The listing builds one solid part. Answer for the finished solid, in the listing's coordinates (mm). Face numbers are marked on the shaded views. A direction names the side the tool comes from. Coordinates: 2 decimals unless noted, no trailing zeros. Loops run counter-clockwise (first coordinate to the right, second up) from the corner with the lowest first, then second, coordinate; pieces in that order, holes last. Notation, with made-up numbers: (74, 23.5) - (133, 23.5) arc R11 ccw to (133, 33.5) - close; hole circle Ø2 at (-15.5, -30.5). An arc over 180 degrees is marked (long way). Return JSON: item names as keys, results as strings. Group by question number.
1. Which of the six approach directions +Z, -Z, +X, -X, +Y, -Y give full straight-line access (tool end or side, diameter ignored) to the marked faces 1 and 2?
2. Find the intervals of material crossed by line 1 along X through (y, z) = (19, -9); line 2 along Y through (x, z) = (2.15, 14.5); line 3 along Y through (x, z) = (-0.75, 16), in increasing order.
3. Section A-A (z = 8) is taken. Write down the section's boundary in (x, y).
4. Section B-B (y = 9.5) is taken. Write down the section's boundary in (x, z).
5. Each of these flat-tipped pins is pushed along its axis until it touches: P1, Ø9, axis at y = 10, z = 2.5, coming from the +X side; P2, Ø0.5, axis at x = -0.5, z = 4, coming from the +Y side; P3, Ø3, axis at y = 18, z = 15, coming from the -X side. Where does it stop, or does it pass through?
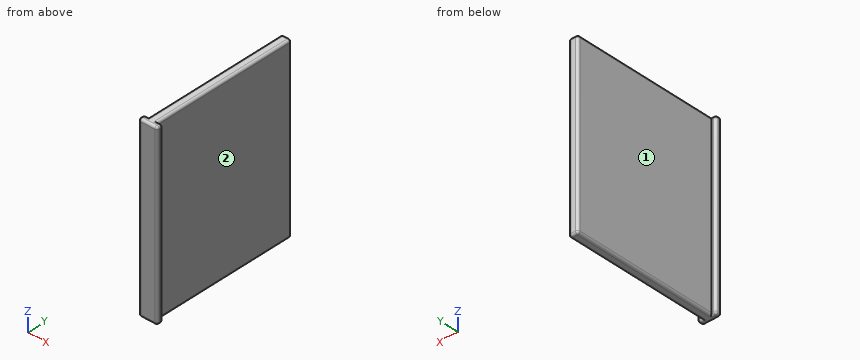
Autodesk Inventor part; units mm, degrees
ref_plane "YZ Plane" through (0, 0, 0) normal (1, 0, 0) x (0, 1, 0)
ref_plane "XZ Plane" through (0, 0, 0) normal (0, 1, 0) x (-1, 0, 0)
ref_plane "XY Plane" through (0, 0, 0) normal (0, 0, 1) x (1, 0, 0)
sketch "Sketch1" plane through (0, 0, 0) normal (0, 0, 1) x (1, 0, 0)
  line L0 (3, 0.8) -> (3, -0.5)
  line L1 (3, -0.5) -> (-1, -0.5)
  line L2 (-1, -0.5) -> (-1, 0.8)
  line L3 (0, 0.8) -> (0, 31.8088)
  line L4 (0, 31.8088) -> (2, 31.8088)
  line L5 (2, 31.8088) -> (2, 0.8)
  line L6 (-1, 0.8) -> (0, 0.8)
  line L7 (2, 0.8) -> (3, 0.8)
  line L8 (-1, 0.8) -> (0, 0.8)
  line L9 (2, 0.8) -> (2.5, 0.8)
  point P0 (0, 0)
  point P1 (1, -0.5)
  point P2 (1, -0.5)
  dimension "d0" = 32.3088
  dimension "d1" = 4
  dimension "d2" = 1.3
  dimension "d3" = 1
  dimension "d4" = 1
extrude "Extrusion1" add sketch "Sketch1" along normal mid plane 37.9984
fillet "Fillet1" radius 0.508 22 edges at (2, 16.3044, 18.9992) (2, 31.8088, 0) (2, 16.3044, -18.9992) (2.5, 0.8, 18.9992) (-0.5, 0.8, 18.9992) (-1, 0.15, 18.9992) (1, -0.5, 18.9992) (3, 0.15, 18.9992) (3, 0.8, 0) (1, 31.8088, 18.9992) (0, 16.3044, 18.9992) (0, 31.8088, 0) (2.5, 0.8, -18.9992) (3, 0.15, -18.9992) (-0.5, 0.8, -18.9992) (-1, 0.15, -18.9992) (1, -0.5, -18.9992) (-1, 0.8, 0) (-1, -0.5, 0) (1, 31.8088, -18.9992) (3, -0.5, 0) (0, 16.3044, -18.9992)
equation "\"d4\" = d3"
properties part number "Tall Conveyor Belt Inserts" material "Acetal Resin, White"
The answers:
{
 "1": {"face 1": "+Z, -Z, -X, +Y", "face 2": "+Z, -Z, +X, +Y"},
 "2": {"line 1": "x = 0 to 2", "line 2": "y = -0.5 to 0.8", "line 3": "y = -0.43 to 0.73"},
 "3": {"outline": "(-1, 0.01) arc R0.51 ccw to (-0.49, -0.5) - (2.49, -0.5) arc R0.51 ccw to (3, 0.01) - (3, 0.29) arc R0.51 ccw to (2.49, 0.8) - (2, 0.8) - (2, 31.3) arc R0.51 ccw to (1.49, 31.81) - (0.51, 31.81) arc R0.51 ccw to (0, 31.3) - (0, 0.8) - (-0.49, 0.8) arc R0.51 ccw to (-1, 0.29) - close"},
 "4": {"outline": "(0, -18.49) arc R0.51 ccw to (0.51, -19) - (1.49, -19) arc R0.51 ccw to (2, -18.49) - (2, 18.49) arc R0.51 ccw to (1.49, 19) - (0.51, 19) arc R0.51 ccw to (0, 18.49) - close"},
 "5": {"P1": "stops at x = 2", "P2": "stops at y = 0.8", "P3": "stops at x = 0"}
}
